Autodesk Inventor part; units mm, degrees
ref_plane "YZ Plane" through (0, 0, 0) normal (1, 0, 0) x (0, 1, 0)
ref_plane "XZ Plane" through (0, 0, 0) normal (0, 1, 0) x (-1, 0, 0)
ref_plane "XY Plane" through (0, 0, 0) normal (0, 0, 1) x (1, 0, 0)
sketch "Sketch1" plane through (0, 0, 0) normal (1, 0, 0) x (0, 1, 0)
  circle A0 centre (0, 0) radius 12
  circle A1 centre (0, -30) radius 12
  line L0 (17, -30) -> (17, 0)
  arc A2 (-17, -30) -> (17, -30) centre (0, -30) ccw
  line L1 (-17, -30) -> (-17, 12)
  line L2 (17, 12) -> (17, 0)
  line L3 (17, 12) -> (17, 17)
  line L4 (17, 17) -> (-17, 17)
  line L5 (-17, 17) -> (-17, 12)
extrude "Extrusion1" add sketch "Sketch1" along normal blind 4
properties part number "lamp_holder_front"
The listing builds one solid part. Answer for the finished solid, in the listing's coordinates (mm). Give positions to 0.01 mm unless a question says otherwise; leave off trailing zeros. Write each loop counter-clockwise with the first axis right and the second up, starting at its lowest first coordinate (ties: lowest second). Pieces come first, ordered by that corner, then holes. Notation, with made-up numbers: (-21, -26.5) - (29, -26.5) arc R26 cw to (29, 6.5) - close; hole circle Ø11 at (80, 44.5). An arc over 180 degrees is marked (long way). Use one line per item in the form item = value. Start each with the question number.
1) Find section D-D on y = 6. Determine the outline of the cut face in (x, z).
2) Find section A-A on z = 0. Determine the outline of the cut face in (x, y), plus the area to 3 significant figures.
3) Find section C-C on x = 2.05. Determine the outline of the cut face in (y, z), plus the area to 3 significant figures.
4) The mould has two halves that part along Y. Classify faces 1 (the face through (2, 0, 17)), 2 (the face through (2, -17, -6)), 3 (the face through (1.97, -11.99, -30.53)): pulls with the +Y half, pulls with the -Y half, needs draft (parallel to the pull), parting line crosses it, or undercut.
5) Find section B-B on y = 0. Determine the outline of the cut face in (x, z), plus the area to 3 significant figures.
6) Consider line 1 along Z through (x, y) = (2, 0); line 2 along Z through (x, y) = (3.7, -5); line 3 along Y through (x, z) = (0.55, -24). Determine where each line is inside the solid, lowest interval first. Write a range as from..to.
7) A flat-ended cylindrical pin translates along its axis: pin 1 Ø1 at (x, z) = (1, -35) entering from -Y. Find the tip coordinate at first contact, or state that the pin passes through.
Geometry results:
q1.outline = (0, -45.91) - (4, -45.91) - (4, -40.39) - (0, -40.39) - close; (0, -19.61) - (4, -19.61) - (4, -10.39) - (0, -10.39) - close; (0, 10.39) - (4, 10.39) - (4, 17) - (0, 17) - close
q2.outline = (0, -17) - (4, -17) - (4, -12) - (0, -12) - close; (0, 12) - (4, 12) - (4, 17) - (0, 17) - close
q2.area = 40.0 mm2
q3.outline = (-17, -30) arc R17 ccw to (17, -30) - (17, 17) - (-17, 17) - close; hole circle Ø24 at (0, -30); hole circle Ø24 at (0, 0)
q3.area = 1,150 mm2
q4.face_1 = needs draft
q4.face_2 = pulls with the -Y half
q4.face_3 = undercut
q5.outline = (0, -47) - (4, -47) - (4, -42) - (0, -42) - close; (0, -18) - (4, -18) - (4, -12) - (0, -12) - close; (0, 12) - (4, 12) - (4, 17) - (0, 17) - close
q5.area = 64.0 mm2
q6.line_1 = -47..-42, -18..-12, 12..17
q6.line_2 = -46.25..-40.91, -19.09..-10.91, 10.91..17
q6.line_3 = -17..-10.39, 10.39..17
q7.pin_1 = -16.39
